Source: three-view drawing plus pictorial views. Frame: mm from the lowest corner of the part. Give positions to 0.01 mm unless a question says otherwise; leave off trailing zeros. Loops run counter-clockwise (first coordinate to the right, second up) from the corner with the lowest first, then second, coordinate; pieces in that order, holes last. Notation, with made-up numbers: (0.25, -3.5) -> (22.25, -3.5) arc R20 ccw to (22.25, 10.5) -> close; hole circle Ø2 at (27.5, -21). An arc over 180 degrees is marked (long way). Put each result on its own line as item: value.
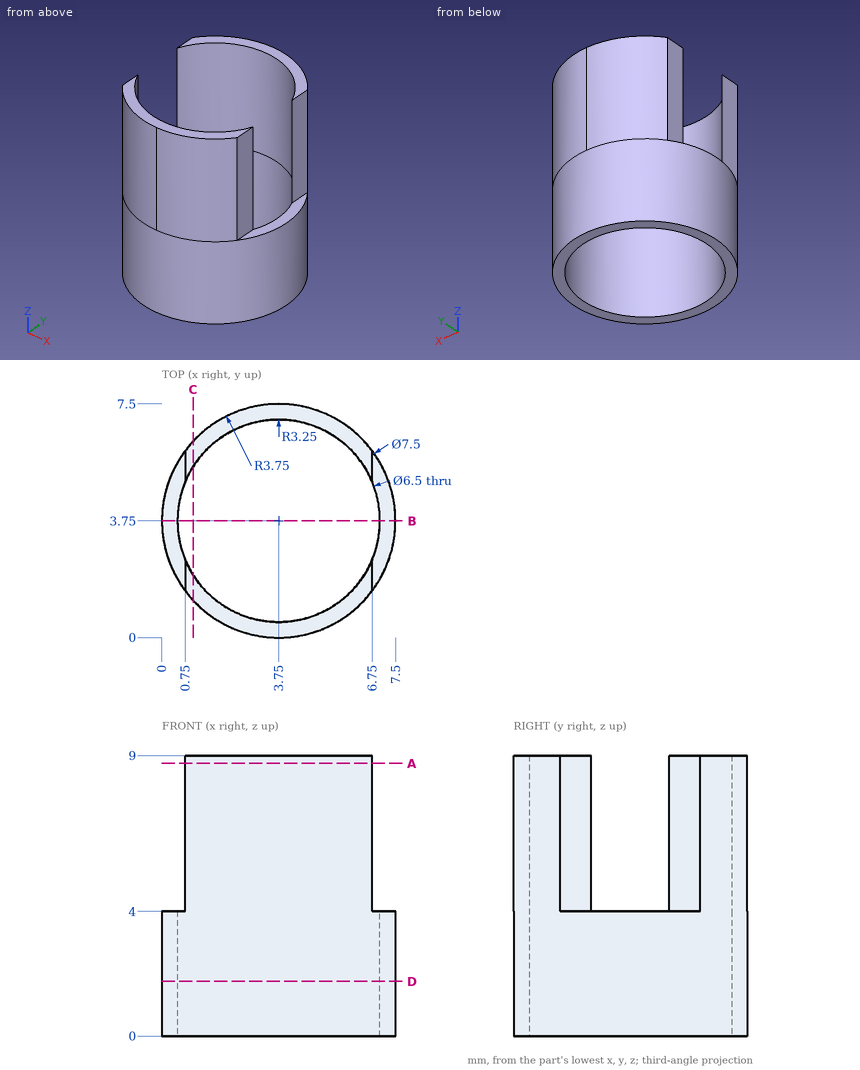
(1) Section B-B on y = 3.75. Return loops of the section in (x, z).
Calculated:
outline: (0, 0) -> (0.5, 0) -> (0.5, 4) -> (0, 4) -> close; (7, 0) -> (7.5, 0) -> (7.5, 4) -> (7, 4) -> close
(2) Section A-A on z = 8.75. Return loops of the section in (x, y).
Calculated:
outline: (0.75, 1.5) arc R3.75 ccw to (6.75, 1.5) -> (6.75, 2.5) arc R3.25 cw to (0.75, 2.5) -> close; (0.75, 5) arc R3.25 cw to (6.75, 5) -> (6.75, 6) arc R3.75 ccw to (0.75, 6) -> close
(3) First-contact query: P1, Ø0.8, axis at y = 5.5, z = 6.5, coming from the -X side; P2, Ø1.1, axis at y = 2, z = 5.5, coming from the -X side; P3, Ø0.6, axis at x = 7, y = 4.5, coming from the +Z side. Flat tips, straight axial feed; report the tip coordinate or a pass-through.
Calculated:
P1: stops at x = 0.75
P2: stops at x = 0.75
P3: stops at z = 4
(4) Line query: probe 1 along Y at (x, z) = (3.75, 5.25); probe 2 along Y at (x, z) = (2, 5.25). Output: solid intervals per line, ascending. Write a range as from..to.
Calculated:
probe 1: y = 0..0.5, 7..7.5
probe 2: y = 0.43..1.01, 6.49..7.07
(5) Section C-C on x = 1. Return loops of the section in (y, z), then the cut area to 3 significant figures.
Calculated:
outline: (1.2, 0) -> (2.02, 0) -> (2.02, 9) -> (1.2, 9) -> close; (5.48, 0) -> (6.3, 0) -> (6.3, 9) -> (5.48, 9) -> close
area: 14.7 mm²
(6) Section D-D on z = 1.75. Return loops of the section in (x, y), then the cut area to 3 significant figures.
Calculated:
outline: circle Ø7.5 at (3.75, 3.75); hole circle Ø6.5 at (3.75, 3.75)
area: 11.0 mm²
